from build123d import *

# Parameters (mm, degrees)
BOSS_EXTRUDE1_DEPTH        = 350
F_6_0_204_DIAMETER_HOLE2_D = 5.1816
F_6_0_204_DIAMETER_HOLE3_D = 5.1816


with BuildPart() as part:
    # Sketch1 → Boss-Extrude1 (new body)
    with BuildSketch(Plane(origin=(0, 0, 0), x_dir=(1, 0, 0), z_dir=(0, 1, 0))):
        Polygon((0, 0), (0, 10), (2, 10), (2, 2), (10, 2), (10, 0), align=None)
    extrude(amount=BOSS_EXTRUDE1_DEPTH)

    # #6 (0.204) Diameter Hole2 (through all)
    with Locations(Plane.ZY):
        with Locations((-5, 5)):
            Hole(F_6_0_204_DIAMETER_HOLE2_D / 2)

    # #6 (0.204) Diameter Hole3 (through all)
    with Locations(Plane.XY):
        with Locations((5, 345)):
            Hole(F_6_0_204_DIAMETER_HOLE3_D / 2)


solid = part.part
The model under review builds one solid part; all positions refer to its coordinate system, in mm. A direction names the side the tool comes from. Give positions to 0.01 mm unless a question says otherwise; leave off trailing zeros. Order: outer loops, then holes, each group sorted by start corner. A loop starts at its lowest first (then second) coordinate and runs counter-clockwise, first axis right, second up. Notation, with made-up numbers: (38, -25) -> (58, -25) arc R18 ccw to (58, 0) -> close; hole circle Ø3 at (-27.5, 66.25). An arc over 180 degrees is marked (long way). Write item = value, one per line. Start each with the question number.
(1) Tool access review of faces 1 (the flat face through (2, 173, -6)), 2 (the flat face through (1.7, 350, -2.8)): name each direction out of +Z, -Z, +X, -X, +Y, -Y from which nothing blocks a thin tool from reaching the whole face with its end or side.
(2) Take a section at A-A (z = -5). Write out the cut boundary in (x, y).
(3) For pin 1 Ø2.5 at (x, y) = (4.5, 161.5) entering from -Z; pin 2 Ø5 at (y, z) = (88, -5) entering from +X, all flat-tipped, find the tip position at first contact; note any pin that passes through.
(4) Take a section at C-C (y = 233.5). Write out the cut boundary in (x, z).
(5) Take a section at B-B (x = 5.75). Write out the cut boundary in (y, z), plus the area to 3 significant figures.
(6) For L1, parallel to Y at x = 5, z = -0.5; L2, parallel to Y at x = 0.65, z = -5; L3, parallel to Z at x = 7, y = 114.5, list the stretches that pass through material, from the lowest coordinate up. Write a range as from..to.
Returned:
q1.face_1 = -Z, +X, +Y, -Y
q1.face_2 = +Z, -Z, +X, -X, +Y
q2.outline = (0, 0) -> (2, 0) -> (2, 2.41) -> (0, 2.41) -> close; (0, 7.59) -> (2, 7.59) -> (2, 350) -> (0, 350) -> close
q3.pin_1 = -2
q3.pin_2 = 2
q4.outline = (0, -10) -> (2, -10) -> (2, -2) -> (10, -2) -> (10, 0) -> (0, 0) -> close
q5.outline = (0, -2) -> (342.52, -2) -> (342.52, 0) -> (0, 0) -> close; (347.48, -2) -> (350, -2) -> (350, 0) -> (347.48, 0) -> close
q5.area = 690 mm²
q6.L1 = 0..342.41, 347.59..350
q6.L2 = 0..2.41, 7.59..350
q6.L3 = -2..0
